from build123d import *

# Parameters (mm, degrees)
F0_R     = 2
F1_DEPTH = 16
F2_R     = 3.5
F3_DEPTH = 4
F5_DEPTH = 3
F6_SIZE  = 0.6


with BuildPart() as f1:
    # F0 (on Right) → F1 (new body)
    with BuildSketch(Plane.YZ):
        Circle(F0_R)
    extrude(amount=-F1_DEPTH)

    # F2 (on face) → F3 (join)
    with BuildSketch(Plane.YZ):
        Circle(F2_R)
    extrude(amount=F3_DEPTH)

    # F4 (on face) → F5 (cut)
    with BuildSketch(Plane.YZ.offset(4)):
        Polygon((1.5, 0.866025), (0, 1.732051), (-1.5, 0.866025), (-1.5, -0.866025), (0, -1.732051), (1.5, -0.866025), align=None)
    extrude(amount=-F5_DEPTH, mode=Mode.SUBTRACT)

    # F6
    f6_edges = [f1.edges().sort_by_distance(p)[0] for p in [
        (-16, -2, 0),
    ]]
    chamfer(f6_edges, length=F6_SIZE)


solid = f1.part
Source: CAD feature listing. Evaluate the final solid. Frame: model axes, mm. A direction names the side the tool comes from. Round coordinates to 2 decimals unless told otherwise and drop trailing zeros. Loops run counter-clockwise (first coordinate to the right, second up) from the corner with the lowest first, then second, coordinate; pieces in that order, holes last. Notation, with made-up numbers: (-33.5, 27.5) - (-13.5, 27.5) arc R19 ccw to (-13.5, 60.5) - close; hole circle Ø9 at (-11.5, -23.5). An arc over 180 degrees is marked (long way). Write item = value, one per line. Start each with the question number.
(1) Pull-direction query (Z, two-part tool) for faces 1 (the face through (1.972, 3.233, -1.341)), 2 (the face through (-16, 0, 0)), 3 (the face through (1, 0, 0)), 4 (the face through (2.521, -0.74, 1.305)); classes: +Z half, -Z half, draft (parallel to the pull), parting line (faces both ways), or undercut.
(2) Ray query, line 1 along X through (y, z) = (1.75, -2); line 2 along Z through (x, y) = (3.25, 1.25); line 3 along Y through (x, z) = (-3, 1). Return the intervals inside material, ascending. Write a range as from..to.
(3) Set-up query: faces 5 (the face through (4, 2, 0)), 6 (the face through (2.521, 0.76, 1.293)), 7 (the face through (0, 2, -2)). Return all of +Z, -Z, +X, -X, +Y, -Y with unobstructed straight access to the full face (end or side cutting, diameter ignored); none if empty.
(4) Section query A-A, the plane z = 0. Output: boundary loops of the cut face in (x, y), plus the area to 3 significant figures.
(5) Pin query (flat end, axial travel): pin 1 (2 mm diameter, centred on x = 0.5, y = -1.5, fed in from -Z); pin 2 (0.9 mm diameter, centred on y = -0.5, z = 0.5, fed in from +X); pin 3 (1 mm diameter, centred on y = 1.5, z = 2.5, fed in from -X). Return the tip coordinate at first contact, or that it passes through.
(6) Section query C-C, the plane y = 3. Output: boundary loops of the cut face in (x, z).
(7) Section query B-B, the plane x = -10. Output: boundary loops of the cut face in (y, z), plus the area to 3 significant figures.
Conclusion:
q1.face_1 = parting line
q1.face_2 = draft
q1.face_3 = undercut
q1.face_4 = undercut
q2.line_1 = 0..4
q2.line_2 = -3.27..-1.01, 1.01..3.27
q2.line_3 = -1.73..1.73
q3.face_5 = +Z, -Z, +X, +Y, -Y
q3.face_6 = +X
q3.face_7 = -X
q4.outline = (-16, -1.4) - (-15.4, -2) - (0, -2) - (0, -3.5) - (4, -3.5) - (4, -1.5) - (1, -1.5) - (1, 1.5) - (4, 1.5) - (4, 3.5) - (0, 3.5) - (0, 2) - (-15.4, 2) - (-16, 1.4) - close
q4.area = 82.6 mm2
q5.pin_1 = -3.46
q5.pin_2 = 1
q5.pin_3 = 0
q6.outline = (0, -1.8) - (4, -1.8) - (4, 1.8) - (0, 1.8) - close
q7.outline = circle Ø4 at (0, 0)
q7.area = 12.6 mm2
